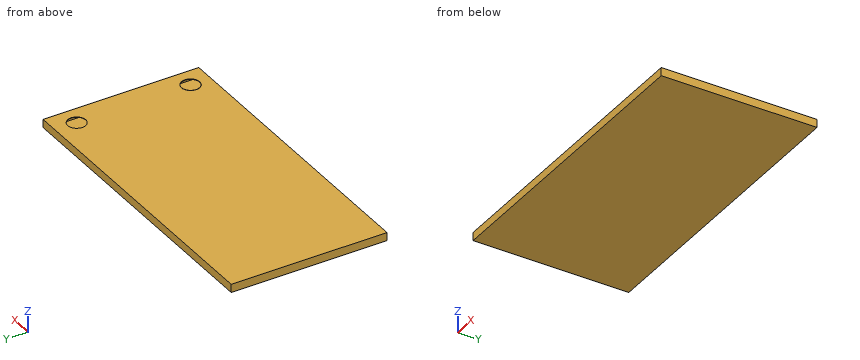
```python
from build123d import *

# Parameters (mm, degrees)
F0_W     = 2040
F0_H     = 1040
F1_DEPTH = 50
F2_W     = 2040
F2_H     = 1040
F2_R     = 60
F3_DEPTH = 2.5
F4_W     = 2040
F4_H     = 1040
F5_DEPTH = 2.5
F6_R     = 61.25
F6_R_2   = 60
F7_DEPTH = 0.5


with BuildPart() as f1:
    # F0 (on Top) → F1 (new body)
    with BuildSketch(Plane.XY):
        Rectangle(F0_W, F0_H)
        Polygon((-1000, 250), (-1000, 500), (-750, 500), (1000, 500), (1000, 497.5), (1000, 250), (1000, -2.028e-07), (1000, -250), (1000, -497.5), (1000, -500), (-750, -500), (-1000, -500), (-1000, -250.0000003493), align=None, mode=Mode.SUBTRACT)
        with BuildLine():
            ThreePointArc((-750, -500), (-926.7766951731, -426.7766954201), (-1000, -250.0000003493))
            Line((-1000, -250.0000003493), (-1000, -500))
            Line((-1000, -500), (-750, -500))
        make_face()
        with BuildLine():
            ThreePointArc((-750, 0), (-926.7766952966, 73.2233047034), (-1000, 250))
            Line((-1000, 250), (-1000, -250.0000003493))
            ThreePointArc((-1000, -250.0000003493), (-926.7766954201, -73.2233048269), (-750, 0))
        make_face()
        with BuildLine():
            Line((-750, 500), (-1000, 500))
            Line((-1000, 500), (-1000, 250))
            ThreePointArc((-1000, 250), (-926.7766952966, 426.7766952966), (-750, 500))
        make_face()
        with BuildLine():
            Line((1000, -2.028e-07), (1000, 250))
            Line((1000, 250), (750, 250))
            ThreePointArc((750, 250), (926.7766953683, 176.7766952249), (1000, -2.028e-07))
        make_face()
        with BuildLine():
            Line((1000, -250), (1000, -2.028e-07))
            ThreePointArc((1000, -2.028e-07), (926.7766952249, -176.7766953683), (750, -250))
            Line((750, -250), (1000, -250))
        make_face()
        with BuildLine():
            ThreePointArc((750, -250), (926.7766952249, -176.7766953683), (1000, -2.028e-07))
            ThreePointArc((1000, -2.028e-07), (926.7766953683, 176.7766952249), (750, 250))
            Line((750, 250), (-750, 250))
            Line((-750, 250), (-750, 247.48))
            Line((-750, 247.48), (746.8536370203, 247.48))
            ThreePointArc((746.8536370203, 247.48), (997.4949999495, 1.5732132723), (750, -247.5))
            Line((750, -247.5), (-750, -247.5))
            Line((-750, -247.5), (-750, -250))
            Line((-750, -250), (750, -250))
        make_face()
        with BuildLine():
            Line((1000, 500), (-750, 500))
            ThreePointArc((-750, 500), (-926.7766952966, 426.7766952966), (-1000, 250))
            ThreePointArc((-1000, 250), (-926.7766952966, 73.2233047034), (-750, 0))
            ThreePointArc((-750, 0), (-926.7766954201, -73.2233048269), (-1000, -250.0000003493))
            ThreePointArc((-1000, -250.0000003493), (-926.7766951731, -426.7766954201), (-750, -500))
            Line((-750, -500), (1000, -500))
            Line((1000, -500), (1000, -497.5))
            Line((1000, -497.5), (-750, -497.5))
            ThreePointArc((-750, -497.5), (-997.5, -250), (-750, -2.5))
            Line((-750, -2.5), (750, -2.5))
            Line((750, -2.5), (750, 2.5))
            Line((750, 2.5), (-750, 2.5))
            ThreePointArc((-750, 2.5), (-997.5, 250), (-750, 497.5))
            Line((-750, 497.5), (1000, 497.5))
            Line((1000, 497.5), (1000, 500))
        make_face()
    extrude(amount=F1_DEPTH)

    # F2 (on face) → F3 (join)
    with BuildSketch(Plane.XY.offset(50)):
        Rectangle(F2_W, F2_H)
        with Locations((890, -385)):
            Circle(F2_R, mode=Mode.SUBTRACT)
        with Locations((890, 375)):
            Circle(F2_R, mode=Mode.SUBTRACT)
    extrude(amount=F3_DEPTH)

    # F4 (on face) → F5 (join)
    with BuildSketch(Plane(origin=(0, 0, 0), x_dir=(1, 0, 0), z_dir=(0, 0, -1))):
        Rectangle(F4_W, F4_H)
    extrude(amount=F5_DEPTH)

    # F6 (on face) → F7 (join)
    with BuildSketch(Plane.XY.offset(52.5)):
        with Locations((890, -385)):
            Circle(F6_R)
        with Locations((890, -385)):
            Circle(F6_R_2, mode=Mode.SUBTRACT)
    extrude(amount=F7_DEPTH)


solid = f1.part
```
Model file for the job. Use its own axes, mm. Coordinates: 2 decimals unless noted, no trailing zeros. Write each loop counter-clockwise with the first axis right and the second up, starting at its lowest first coordinate (ties: lowest second). Pieces come first, ordered by that corner, then holes. Notation, with made-up numbers: (1, 39) - (25, 39) arc R23 cw to (25, 48) - close; hole circle Ø9 at (29, 32.5). An arc over 180 degrees is marked (long way). One line per item, written item: value. Start each with the question number.
1. Slice it at B-B (x = -134). Write the cut outline in (y, z), plus the area to 3 significant figures.
2. Slice it at D-D (x = 890). Write the cut outline in (y, z).
3. Probe line 1 (Y direction, x = -72, z = 1); line 2 (Y direction, x = 890, z = 51); line 3 (Z direction, x = -585, y = -65). List the from-to ranges inside material, lowest first. Write a range as from..to.
4. Slice it at A-A (z = 9). Write the cut outline in (x, y).
5. Slice it at C-C (y = -205.5). Write the cut outline in (x, z), plus the area to 3 significant figures.
6. Flat gauge pin, fed straight in: pin 1 (10 mm diameter, centred on x = -585, y = -3.5, fed in from +Z). Where does the tip first touch, or does it go through?
Answers below:
1. outline: (-520, -2.5) - (520, -2.5) - (520, 52.5) - (-520, 52.5) - close; hole (-497.5, 0) - (-250, 0) - (-250, 50) - (-497.5, 50) - close; hole (-247.5, 0) - (-2.5, 0) - (-2.5, 50) - (-247.5, 50) - close; hole (2.5, 0) - (247.48, 0) - (247.48, 50) - (2.5, 50) - close; hole (250, 0) - (497.5, 0) - (497.5, 50) - (250, 50) - close
1. area: 7,950 mm^2
2. outline: (-520, -2.5) - (520, -2.5) - (520, 52.5) - (435, 52.5) - (435, 50) - (497.5, 50) - (497.5, 0) - (250, 0) - (250, 50) - (315, 50) - (315, 52.5) - (-323.75, 52.5) - (-323.75, 53) - (-325, 53) - (-325, 50) - (-250, 50) - (-250, 0) - (-497.5, 0) - (-497.5, 50) - (-445, 50) - (-445, 53) - (-446.25, 53) - (-446.25, 52.5) - (-520, 52.5) - close; hole (-204.1, 0) - (204.1, 0) - (204.1, 50) - (-204.1, 50) - close
3. line 1: y = -520..-497.5, -250..-247.5, -2.5..2.5, 247.48..250, 497.5..520
3. line 2: y = -520..-445, -325..315, 435..520
3. line 3: z = -2.5..0, 50..52.5
4. outline: (-1020, -520) - (1020, -520) - (1020, 520) - (-1020, 520) - close; hole (-750, -497.5) - (1000, -497.5) - (1000, -250) - (-750, -250) - (-750, -247.5) - (750, -247.5) arc R247.5 ccw (long way) to (746.85, 247.48) - (-750, 247.48) - (-750, 250) - (1000, 250) - (1000, 497.5) - (-750, 497.5) arc R247.5 ccw to (-750, 2.5) - (750, 2.5) - (750, -2.5) - (-750, -2.5) arc R247.5 ccw to start
5. outline: (-1020, -2.5) - (1020, -2.5) - (1020, 52.5) - (-1020, 52.5) - close; hole (-993.47, 0) - (887.93, 0) - (887.93, 50) - (-993.47, 50) - close
5. area: 18,100 mm^2
6. pin 1: stops at z = 52.5
